Geometry check sheet. Reference: the model listing, model coordinates, mm. A direction names the side the tool comes from. Round coordinates to 2 decimals unless told otherwise and drop trailing zeros. Order: outer loops, then holes, each group sorted by start corner. A loop starts at its lowest first (then second) coordinate and runs counter-clockwise, first axis right, second up. Notation, with made-up numbers: M 52,-7.75 L 100,-7.75 A24 cw 100,23.25 Z; hole C 68.5,44 d4. An arc over 180 degrees is marked long. Return JSON: item names as keys, results as strings. Group by question number.
```python
from build123d import *

# Parameters (mm, degrees)
F0_W     = 38.1
F0_H     = 50.8
F1_DEPTH = 38.1
F2_T     = -2.54
F4_DEPTH = 25.4


with BuildPart() as f1:
    # F0 (on Front) → F1 (new body)
    with BuildSketch(Plane.XZ):
        with Locations((-47.1864644898, 25.4)):
            Rectangle(F0_W, F0_H)
        with BuildLine():
            ThreePointArc((-28.1364644898, 50.8), (-47.1864644898, 69.85), (-66.2364644898, 50.8))
            Line((-66.2364644898, 50.8), (-28.1364644898, 50.8))
        make_face()
    extrude(amount=F1_DEPTH)

    # F2 (hollow: no face is removed)
    offset(amount=F2_T, mode=Mode.SUBTRACT)

    # F3 (on face) → F4 (cut)
    with BuildSketch(Plane.XZ.offset(38.1)):
        with BuildLine():
            ThreePointArc((-42.1064644898, 59.055), (-42.8504132656, 60.8510512242), (-44.6464644898, 61.595))
            Line((-44.6464644898, 61.595), (-49.7264644898, 61.595))
            ThreePointArc((-49.7264644898, 61.595), (-51.522515714, 60.8510512242), (-52.2664644898, 59.055))
            Line((-52.2664644898, 59.055), (-52.2664644898, 10.795))
            ThreePointArc((-52.2664644898, 10.795), (-51.522515714, 8.9989487758), (-49.7264644898, 8.255))
            Line((-49.7264644898, 8.255), (-44.6464644898, 8.255))
            ThreePointArc((-44.6464644898, 8.255), (-42.8504132656, 8.9989487758), (-42.1064644898, 10.795))
            Line((-42.1064644898, 10.795), (-42.1064644898, 59.055))
        make_face()
    extrude(amount=-F4_DEPTH, mode=Mode.SUBTRACT)


solid = f1.part
```
Q1. Section check A-A on y = -27.5. Record the cut outline in (x, z).
Q2. Section check D-D on x = -37. Record the cut outline in (y, z), plus the area to 3 significant figures.
Q3. Material ranges on line 1 along Y through (x, z) = (-56.5, 11); line 2 along X through (y, z) = (-20, 48); line 3 along Y through (x, z) = (-49, 35), recorded low to high.
Q4. Section check B-B on z = 17. Record the cut outline in (x, y).
Q5. Set-up check for faces 1 (the face through (-46.768, -18.783, 69.845)), 2 (the face through (-47, -19, 2.54)), 3 (the face through (-47, -37, 61.595)): record each of +Z, -Z, +X, -X, +Y, -Y from which the full face is reachable in a straight line by a thin tool's end or side.
Q6. Release check for a two-part mould opening along X. For faces 4 (the face through (-51.503, -36.848, 60.871)), 5 (the face through (-47, 0, 35)), 6 (the face through (-66.236, -19, 25)) record: +X half, -X half, draft (parallel to the pull), parting line (faces both ways), or undercut.
Q7. Depth check by flat-ended pin: pin 1 Ø5 at (x, y) = (-62.5, -25) entering from +Z; pin 2 Ø3 at (x, y) = (-49, -8) entering from +Z; pin 3 Ø3 at (x, y) = (-58, -19) entering from +Z. Enter the tip coordinate at first touch or a pass-through.
Q8. Section check C-C on x = -43.5. Record the cut outline in (y, z).
Geometry check:
{
 "1": {"outline": "M -66.24,0 L -28.14,0 L -28.14,50.8 A19.05 ccw -66.24,50.8 Z; hole M -63.7,2.54 L -30.68,2.54 L -30.68,50.8 A16.51 ccw -63.7,50.8 Z"},
 "2": {"outline": "M -38.1,0 L 0,0 L 0,66.9 L -38.1,66.9 Z; hole M -35.56,2.54 L -2.54,2.54 L -2.54,63.79 L -35.56,63.79 Z", "area": "526 mm^2"},
 "3": {"line 1": "y = -38.1 to -35.56, -2.54 to 0", "line 2": "x = -66.24 to -63.7, -30.68 to -28.14", "line 3": "y = -2.54 to 0"},
 "4": {"outline": "M -66.24,-38.1 L -52.27,-38.1 L -52.27,-35.56 L -63.7,-35.56 L -63.7,-2.54 L -30.68,-2.54 L -30.68,-35.56 L -42.11,-35.56 L -42.11,-38.1 L -28.14,-38.1 L -28.14,0 L -66.24,0 Z"},
 "5": {"face 1": "+Z, +Y, -Y", "face 2": "none", "face 3": "-Y"},
 "6": {"face 4": "undercut", "face 5": "draft", "face 6": "-X half"},
 "7": {"pin 1": "stops at z = 64.9", "pin 2": "stops at z = 69.85", "pin 3": "stops at z = 67.42"},
 "8": {"outline": "M -38.1,0 L 0,0 L 0,69.49 L -38.1,69.49 L -38.1,61.32 L -35.56,61.32 L -35.56,66.89 L -2.54,66.89 L -2.54,2.54 L -35.56,2.54 L -35.56,8.53 L -38.1,8.53 Z"}
}
